from build123d import *

# Parameters (mm, degrees)
SKETCH1_R           = 127
BOSS_EXTRUDE1_DEPTH = 3.175
SKETCH2_W           = 12.438745875
SKETCH2_H           = 31.000011437
CUT_EXTRUDE1_DEPTH  = 3.175


with BuildPart() as part:
    # Sketch1 → Boss-Extrude1 (new body)
    with BuildSketch(Plane(origin=(0, 0, 0), x_dir=(1, 0, 0), z_dir=(0, 1, 0))):
        with Locations(Location((0, 0, 0), (0, 0, 270))):
            Circle(SKETCH1_R)
    extrude(amount=BOSS_EXTRUDE1_DEPTH)

    # Sketch2 → Cut-Extrude1 (cut)
    with BuildSketch(Plane(origin=(0, 3.175, 0), x_dir=(1, 0, 0), z_dir=(0, 1, 0))):
        Polygon((-51.846570392, -27.761273072), (-67.392708125, -27.761273072), (-63.49777994, -32.449612553), (-87.392519872, -68.724363756), (-73.025563352, -68.724363756), (-68.858940519, -62.398988085), (-63.49777994, -53.443146367), (-56.052860633, -41.035320282), (-47.711513929, -53.443146367), (-61.129520895, -53.443146367), (-66.490681474, -62.398988085), (-43.246780748, -62.398988085), (-37.991853267, -68.724363756), (-24.308519881, -68.724363756), align=None)
        with BuildLine():
            Line((47.513174781, -27.761273072), (35.129585086, -27.761273072))
            Line((35.129585086, -27.761273072), (50.616895331, -49.460734396))
            add(Edge.make_bspline(
                [(45.679130911, -46.040196269), (31.550212316, -41.255173944), (28.733398827, -52.539450499), (25.916585337, -63.823727055), (41.797676766, -61.589469293), (57.678768195, -59.355211531), (50.616895331, -49.460734396)],
                knots=[1.020082476, 1.020082476, 1.020082476, 2.907145281, 2.907145281, 4.794208086, 4.794208086, 6.681270891, 6.681270891, 6.681270891], degree=2, weights=[1, 0.586932541, 1, 0.586932541, 1, 0.586932541, 1]))
            Line((45.679130911, -46.040196269), (39.850903677, -37.874195236))
            add(Edge.make_bspline(
                [(39.850903677, -37.874195236), (-30.231497677, -39.73502536), (26.658902193, -66.440769536), (83.549302064, -93.146513713), (62.228166445, -48.37862931)],
                knots=[1.563851242, 1.563851242, 1.563851242, 4.067513609, 4.067513609, 6.571175976, 6.571175976, 6.571175976], degree=2, weights=[1, 0.31358407, 1, 0.31358407, 1]))
            Line((62.228166445, -48.37862931), (47.513174781, -27.761273072))
        make_face()
        with BuildLine():
            Line((-14.629199742, -37.724352319), (-24.813373872, -37.724352319))
            Line((-24.813373872, -37.724352319), (-24.813373872, -59.074478125))
            ThreePointArc((-24.813373872, -59.074478125), (-7.314599871, -68.724363756), (10.184174129, -59.074478125))
            Line((10.184174129, -59.074478125), (10.184174129, -37.724352319))
            Line((10.184174129, -37.724352319), (0, -37.724352319))
            Line((0, -37.724352319), (0, -58.665309043))
            ThreePointArc((0, -58.665309043), (-7.314599871, -61.774148851), (-14.629199742, -58.665309043))
            Line((-14.629199742, -58.665309043), (-14.629199742, -37.724352319))
        make_face()
        with Locations((71.910421643, -53.224358038)):
            Rectangle(SKETCH2_W, SKETCH2_H)
        with BuildLine():
            ThreePointArc((-57.663269864, 57.359209553), (-54.545921341, 60.836930705), (-51.064741507, 63.950416403))
            ThreePointArc((-51.064741507, 63.950416403), (-102.357132874, 2.042968688), (-41.531381183, 54.613582399))
            ThreePointArc((-41.531381183, 54.613582399), (-45.091015331, 51.621496868), (-48.12990954, 48.101739338))
            ThreePointArc((-48.12990954, 48.101739338), (-95.868420767, 8.4780016), (-57.663269864, 57.359209553))
        make_face()
        with BuildLine():
            ThreePointArc((-50.606514106, 13.62018236), (-46.986171072, 52.596169792), (-8.133269864, 57.359209553))
            ThreePointArc((-8.133269864, 57.359209553), (-5.015921341, 60.836930705), (-1.534741507, 63.950416403))
            ThreePointArc((-1.534741507, 63.950416403), (-31.275194817, 70.642250855), (-57.205042464, 54.613582399))
            ThreePointArc((-57.205042464, 54.613582399), (-64.940122856, 30.860960849), (-57.205042464, 7.108339298))
            ThreePointArc((-57.205042464, 7.108339298), (-53.645408316, 10.100424829), (-50.606514106, 13.62018236))
        make_face()
        with BuildLine():
            ThreePointArc((-1.076514106, 13.62018236), (2.543828928, 52.596169792), (41.396730136, 57.359209553))
            ThreePointArc((41.396730136, 57.359209553), (44.514078659, 60.836930705), (47.995258493, 63.950416403))
            ThreePointArc((47.995258493, 63.950416403), (-3.891203984, 59.084881899), (-7.675042464, 7.108339298))
            ThreePointArc((-7.675042464, 7.108339298), (-4.115408316, 10.100424829), (-1.076514106, 13.62018236))
        make_face()
        with BuildLine():
            ThreePointArc((48.453485894, 13.62018236), (96.19199712, 53.243920097), (57.986846218, 4.362712144))
            ThreePointArc((57.986846218, 4.362712144), (54.869497694, 0.884990992), (51.38831786, -2.228494706))
            ThreePointArc((51.38831786, -2.228494706), (102.680709227, 59.678953009), (41.854957536, 7.108339298))
            ThreePointArc((41.854957536, 7.108339298), (45.414591684, 10.100424829), (48.453485894, 13.62018236))
        make_face()
        with BuildLine():
            ThreePointArc((1.40009046, 48.101739338), (-2.220252575, 9.125751905), (-41.073153782, 4.362712144))
            ThreePointArc((-41.073153782, 4.362712144), (-44.190502306, 0.884990992), (-47.67168214, -2.228494706))
            ThreePointArc((-47.67168214, -2.228494706), (4.214780337, 2.637039798), (7.998618817, 54.613582399))
            ThreePointArc((7.998618817, 54.613582399), (4.438984669, 51.621496868), (1.40009046, 48.101739338))
        make_face()
        with BuildLine():
            ThreePointArc((50.93009046, 48.101739338), (47.309747425, 9.125751905), (8.456846218, 4.362712144))
            ThreePointArc((8.456846218, 4.362712144), (5.339497694, 0.884990992), (1.85831786, -2.228494706))
            ThreePointArc((1.85831786, -2.228494706), (53.744780337, 2.637039798), (57.528618817, 54.613582399))
            ThreePointArc((57.528618817, 54.613582399), (53.968984669, 51.621496868), (50.93009046, 48.101739338))
        make_face()
    extrude(amount=-CUT_EXTRUDE1_DEPTH, mode=Mode.SUBTRACT)


solid = part.part
Verification items for the finished model (mm, model axes). Coordinates: 2 decimals unless noted, no trailing zeros. Order: outer loops, then holes, each group sorted by start corner. A loop starts at its lowest first (then second) coordinate and runs counter-clockwise, first axis right, second up. Notation, with made-up numbers: (39, 25.25) -> (58, 25.25) arc R12 ccw to (58, 43.25) -> close; hole circle Ø10 at (37.5, 0.25). An arc over 180 degrees is marked (long way). Put each result on its own line as item: value. Start each with the question number.
1. Cross-section at C-C, the plane x = -101.5. Record the boundary of the cut face in (y, z) (3 decimals).
2. Cross-section at A-A, the plane x = 88.5. Record the boundary of the cut face in (y, z) (1 decimal), then the cut area to 3 significant figures.
3. Cross-section at D-D, the plane z = -96. Record the boundary of the cut face in (x, y) (3 decimals).
4. Mould release check, pull along Z, two halves, no side actions. Record for faces 1 (the cylindrical face through (-44.144, 1.61, -0.931)), 2 (the flat face through (-26, 0, -2)): released by +Z, released by -Z, zero draft, split by the parting line, or undercut.
5. Material ranges on L1, parallel to X at y = 2.75, z = 30; L2, parallel to Z at x = 91, y = 1.4; L3, parallel to Z at x = -42, y = 1, recorded low to high. Write a range as [from, to].
6. Go/stop test with flat-tipped pins: pin 1 Ø1.6 at (x, y) = (-81, 1.5) entering from -Z; pin 2 Ø1.6 at (y, z) = (1, 51.5) entering from +X; pin 3 Ø1 at (x, y) = (-19, 1.5) entering from +Z. Record where each tip stops, or that it passes through.
7. Cross-section at B-B, the plane y = 0.75. Count the separate pieces of the cut face and the enclosed holes in it, then the cut area to 3 significant figures.
Computed:
1. outline: (0, -76.333) -> (3.175, -76.333) -> (3.175, -60.494) -> (0, -60.494) -> close; (0, -45.843) -> (3.175, -45.843) -> (3.175, -15.878) -> (0, -15.878) -> close; (0, -1.228) -> (3.175, -1.228) -> (3.175, 76.333) -> (0, 76.333) -> close
2. outline: (0, -91.1) -> (3.2, -91.1) -> (3.2, -68.7) -> (0, -68.7) -> close; (0, -58.7) -> (3.2, -58.7) -> (3.2, -3) -> (0, -3) -> close; (0, 7) -> (3.2, 7) -> (3.2, 91.1) -> (0, 91.1) -> close
2. area: 515 mm2
3. outline: (-83.144, 0) -> (83.144, 0) -> (83.144, 3.175) -> (-83.144, 3.175) -> close
4. face 1: undercut
4. face 2: zero draft
5. L1: [-123.41, -65.53], [-50.34, 36.73], [49.11, 123.41]
5. L2: [-88.59, -67.65], [-57.31, -4.41], [5.93, 88.59]
5. L3: [-119.85, -67.25], [-56.76, -54.27], [-6.48, -3.25], [5.53, 42.41], [63.9, 119.85]
6. pin 1: z = -98.47
6. pin 2: x = 116.44
6. pin 3: z = 125.65
7. separate pieces: 1
7. enclosed holes: 10
7. area: 40,000 mm2
